from build123d import *

# Parameters (mm, degrees)
CROQUIS1_R           = 16.75
CROQUIS1_R_2         = 14.75
PESTA_AENTRADA_DEPTH = 4.5
CROQUIS2_R           = 27.5
TAPADERA_DEPTH       = 2
DETALLESUPERIOR_R    = 1


with BuildPart() as part:
    # Croquis1 → PestañaEntrada (new body)
    with BuildSketch(Plane.XY):
        Circle(CROQUIS1_R)
        Circle(CROQUIS1_R_2, mode=Mode.SUBTRACT)
    extrude(amount=PESTA_AENTRADA_DEPTH)

    # Croquis2 → Tapadera (add)
    with BuildSketch(Plane(origin=(0, 0, 0), x_dir=(-1, 0, 0), z_dir=(0, 0, -1))):
        Circle(CROQUIS2_R)
    extrude(amount=TAPADERA_DEPTH)

    # DetalleSuperior
    detallesuperior_edges = [part.edges().sort_by_distance(p)[0] for p in [
        (27.5, 0, -2),
    ]]
    fillet(detallesuperior_edges, radius=DETALLESUPERIOR_R)


solid = part.part
Verification items for the finished model (mm, model axes). A direction names the side the tool comes from. Coordinates: 2 decimals unless noted, no trailing zeros. Write each loop counter-clockwise with the first axis right and the second up, starting at its lowest first coordinate (ties: lowest second). Pieces come first, ordered by that corner, then holes. Notation, with made-up numbers: M 15,17.25 L 30,17.25 A29 ccw 30,40.25 Z; hole C 21.25,-7 d9. An arc over 180 degrees is marked long. Use a Markdown table: item, result.
Q1. Thickness scan on line 1 (Y direction, x = 0, z = 3.2); line 2 (Z direction, x = -3.5, y = 3.5); line 3 (Y direction, x = 12.5, z = 0.5). Record the ranges inside material, lowest first.
Reply:
| item | result |
|---|---|
| line 1 | y = -16.75 to -14.75, 14.75 to 16.75 |
| line 2 | z = -2 to 0 |
| line 3 | y = -11.15 to -7.83, 7.83 to 11.15 |
Q2. Sectioned sample at C-C, the plane z = 1.25. Record the boundary of the cut face in (x, y), plus the area to 3 significant figures.
Reply:
| item | result |
|---|---|
| outline | C 0,0 d33.5; hole C 0,0 d29.5 |
| area | 198 mm² |
Q3. Go/stop test with flat-tipped pins: P1, Ø2, axis at y = -14.5, z = 3, coming from the +X side; P2, Ø23.5, axis at x = -2, y = 7, coming from the +Z side; P3, Ø1.5, axis at x = 14, z = 0.5, coming from the +Y side; P4, Ø3, axis at x = 17.5, z = -0.5, coming from the -Y side. Record where each tip stops, or that it passes through.
Reply:
| item | result |
|---|---|
| P1 | stops at x = 9.92 |
| P2 | stops at z = 4.5 |
| P3 | stops at y = 23.99 |
| P4 | stops at y = -22.37 |
Q4. Draft check along Y on faces 3 (the face through (0, 0, 0)), 4 (the face through (0, -15, 4.5)), 5 (the face through (5.961, -26.846, -0.493)). Enter one of: +Y half, -Y half, draft (parallel to the pull), parting line (faces both ways), or undercut.
Reply:
| item | result |
|---|---|
| face 3 | undercut |
| face 4 | draft |
| face 5 | parting line |
Q5. Sectioned sample at A-A, the plane y = 0. Record the boundary of the cut face in (x, z).
Reply:
| item | result |
|---|---|
| outline | M -27.5,-1 A1 ccw -26.5,-2 L 26.5,-2 A1 ccw 27.5,-1 L 27.5,0 L 16.75,0 L 16.75,4.5 L 14.75,4.5 L 14.75,0 L -14.75,0 L -14.75,4.5 L -16.75,4.5 L -16.75,0 L -27.5,0 Z |
Q6. Set-up check for faces 1 (the face through (0, 0, -2)), 2 (the face through (14.07, 4.43, 2.22)): record each of +Z, -Z, +X, -X, +Y, -Y from which the full face is reachable in a straight line by a thin tool's end or side.
Reply:
| item | result |
|---|---|
| face 1 | -Z, +X, -X, +Y, -Y |
| face 2 | +Z |
